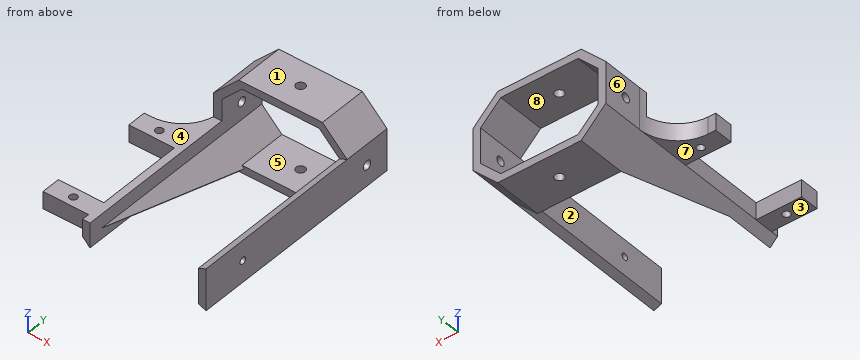
```python
from build123d import *

# Parameters (mm, degrees)
BOSS_EXTRUDE1_DEPTH = 13
BOSS_EXTRUDE2_DEPTH = 46
SKETCH8_R           = 0.9
CUT_EXTRUDE1_DEPTH  = 10
SKETCH9_R           = 1.2
CUT_EXTRUDE2_DEPTH  = 40
SKETCH10_R          = 1.2
CUT_EXTRUDE3_DEPTH  = 50
BOSS_EXTRUDE3_DEPTH = 43
SKETCH12_W          = 4.508561795
SKETCH12_H          = 5
BOSS_EXTRUDE4_DEPTH = 12
SKETCH14_R          = 1
CUT_EXTRUDE4_DEPTH  = 30
BOSS_EXTRUDE5_DEPTH = 2
FILLET3_R           = 10
BOSS_EXTRUDE6_DEPTH = 46
SKETCH8_2_R         = 0.9
CUT_EXTRUDE5_DEPTH  = 30


with BuildPart() as part:
    # Sketch1 → Boss-Extrude1 (new body)
    with BuildSketch(Plane(origin=(0, 0, 0), x_dir=(1, 0, 0), z_dir=(0, 1, 0))):
        Polygon((-7.31986533, -4.491438205), (-0.828427125, 2), (21.188696525, 2), (27.68013467, -4.491438145), (27.68013467, -15.508561795), (21.188696464, -22), (-0.828427125, -22), (-7.31986533, -15.508561795), align=None)
        Polygon((0, 0), (20.3602694, 0), (25.68013467, -5.31986527), (25.68013467, -14.68013467), (20.36026934, -20), (0, -20), (-5.31986533, -14.68013467), (-5.31986533, -5.31986533), align=None, mode=Mode.SUBTRACT)
    extrude(amount=BOSS_EXTRUDE1_DEPTH)

    # Sketch7 → Boss-Extrude2 (add)
    with BuildSketch(Plane.XZ):
        with BuildLine():
            ThreePointArc((27.68013467, 12.696190421), (26.68013467, 13.696190421), (25.68013467, 12.696190421))
            Line((25.68013467, 12.696190421), (25.68013467, 7.303809579))
            ThreePointArc((25.68013467, 7.303809579), (26.68013467, 6.303809579), (27.68013467, 7.303809579))
            Line((27.68013467, 7.303809579), (27.68013467, 12.696190421))
        make_face()
    extrude(amount=BOSS_EXTRUDE2_DEPTH)

    # Sketch8 → Cut-Extrude1 (cut)
    with BuildSketch(Plane(origin=(27.68013467, 0, 0), x_dir=(0, 0, -1), z_dir=(1, 0, 0))):
        with Locations((-10.196190421, -34)):
            Circle(SKETCH8_R)
    extrude(amount=-CUT_EXTRUDE1_DEPTH, mode=Mode.SUBTRACT)

    # Sketch9 → Cut-Extrude2 (cut)
    with BuildSketch(Plane.XY.offset(22)):
        with Locations((10.171572875, 6.5)):
            Circle(SKETCH9_R)
    extrude(amount=-CUT_EXTRUDE2_DEPTH, mode=Mode.SUBTRACT)

    # Sketch10 → Cut-Extrude3 (cut)
    with BuildSketch(Plane(origin=(27.68013467, 0, 0), x_dir=(0, 0, -1), z_dir=(1, 0, 0))):
        with Locations((-10, 6.5)):
            Circle(SKETCH10_R)
    extrude(amount=-CUT_EXTRUDE3_DEPTH, mode=Mode.SUBTRACT)

    # Sketch11 → Boss-Extrude3 (add)
    with BuildSketch(Plane.XZ):
        Polygon((-5.31986533, 9), (-7.31986533, 9), (-7.31986533, 4.491438205), (-5.31986533, 2.491438205), align=None)
    extrude(amount=BOSS_EXTRUDE3_DEPTH)

    # Sketch12 → Boss-Extrude4 (add)
    with BuildSketch(Plane.ZY.offset(7.31986533)):
        with Locations((6.745719103, -10.5)):
            Rectangle(SKETCH12_W, SKETCH12_H)
        with Locations((6.745719103, -38.5)):
            Rectangle(SKETCH12_W, SKETCH12_H)
    extrude(amount=BOSS_EXTRUDE4_DEPTH)

    # Sketch14 → Cut-Extrude4 (cut)
    with BuildSketch(Plane.XY.offset(9)):
        with Locations((-13.31986532, -10.5)):
            Circle(SKETCH14_R)
        with Locations((-13.31986532, -38.5)):
            Circle(SKETCH14_R)
    extrude(amount=-CUT_EXTRUDE4_DEPTH, mode=Mode.SUBTRACT)

    # Sketch17 → Boss-Extrude5 (add)
    with BuildSketch(Plane(origin=(-1.414213562, 0, -1.414213562), x_dir=(-0.7071067811865714, 0, 0.7071067811865236), z_dir=(-0.7071067811865236, 0, -0.7071067811865714))):
        Polygon((-0.828427125, 0), (8.351852825, -43), (8.351852825, 0), align=None)
    extrude(amount=-BOSS_EXTRUDE5_DEPTH)

    # Fillet3
    fillet3_edges = [part.edges().sort_by_distance(p)[0] for p in [
        (-7.31986533, -8, 6.745719103),
    ]]
    fillet(fillet3_edges, radius=FILLET3_R)

    # Sketch18 → Boss-Extrude6 (add)
    with BuildSketch(Plane.XZ):
        Polygon((27.68013467, 15.508561795), (25.68013467, 14.68013467), (25.68013467, 5.31986527), (27.68013467, 4.491438145), align=None)
    extrude(amount=BOSS_EXTRUDE6_DEPTH)

    # Sketch8<2> → Cut-Extrude5 (cut)
    with BuildSketch(Plane(origin=(27.68013467, 0, 0), x_dir=(0, 0, -1), z_dir=(1, 0, 0))):
        with Locations((-10.196190421, -34)):
            Circle(SKETCH8_2_R)
    extrude(amount=-CUT_EXTRUDE5_DEPTH, mode=Mode.SUBTRACT)


solid = part.part
```
Can you work these out from the model? Positions are in its coordinate system, mm. Face numbers are marked on the shaded views. A direction names the side the tool comes from. Give positions to 0.01 mm unless a question says otherwise; leave off trailing zeros. Write each loop counter-clockwise with the first axis right and the second up, starting at its lowest first coordinate (ties: lowest second). Pieces come first, ordered by that corner, then holes. Notation, with made-up numbers: (85.25, -13.5) -> (101.25, -13.5) arc R15 ccw to (101.25, -7.5) -> close; hole circle Ø10 at (-38, 18.25). An arc over 180 degrees is marked (long way). One line per item, written item: value.
Q1. We'd pull the mould along Z, two halves only. Please class the marked faces 5, 6, 7 and 8: +Z half, -Z half, draft (parallel to the pull), parting line (faces both ways), or undercut.
Results found:
face 5: undercut
face 6: draft
face 7: -Z half
face 8: undercut
Q2. Imagine slicing it at B-B on x = 4.5. Please give me the cut outline in (y, z), and give its area (3 significant figures).
Results found:
outline: (0, -2) -> (13, -2) -> (13, 0) -> (0, 0) -> close; (0, 20) -> (13, 20) -> (13, 22) -> (0, 22) -> close
area: 52.0 mm^2
Q3. Imagine slicing it at C-C on z = 17.75. Please give me the cut outline in (x, y).
Results found:
outline: (-5.08, 0) -> (-2.25, 0) -> (-2.25, 13) -> (-5.08, 13) -> close; (22.61, 0) -> (25.44, 0) -> (25.44, 13) -> (22.61, 13) -> close
Q4. Imagine slicing it at D-D on z = 10. Please give me the cut outline in (x, y).
Results found:
outline: (-7.52, 0) -> (-5.32, 0) -> (-5.32, 5.3) -> (-7.32, 5.3) -> (-7.32, 2) arc R10 cw to start; (-7.32, 7.7) -> (-5.32, 7.7) -> (-5.32, 13) -> (-7.32, 13) -> close; (25.68, -46) -> (27.68, -46) -> (27.68, -34.88) -> (25.68, -34.88) -> close; (25.68, -33.12) -> (27.68, -33.12) -> (27.68, 5.3) -> (25.68, 5.3) -> close; (25.68, 7.7) -> (27.68, 7.7) -> (27.68, 13) -> (25.68, 13) -> close
Q5. Which directions (+Z, -Z, +X, -X, +Y, -Y) give clear straight access to the entire face, cutting with the end or side of a thin tool? Please do the marked faces 1, 2, 3 and 4.
Results found:
face 1: +Z, +X, -X, +Y, -Y
face 2: +Y, -Y
face 3: -Z, -X, +Y, -Y
face 4: +Z, -X, -Y
Q6. Please list where these lines run through material, in increasing order: line 1 (X direction, y = -13.5, z = 6.5); line 2 (X direction, y = -3, z = 8.25); line 3 (Z direction, x = -5, y = 6). Write a range as [from, to].
Results found:
line 1: x = [-7.32, -5.32], [25.68, 27.68]
line 2: x = [-8.66, -5.32], [25.68, 27.68]
line 3: z = [2.17, 5], [15, 17.83]
Q7. For P1, Ø3, axis at y = 6.5, z = 10, coming from the -X side; P2, Ø3.5, axis at x = -16, z = 7, coming from the +Y side; P3, Ø1, axis at x = -18.5, z = 6.5, coming from the +Y side; P4, Ø3, axis at x = 20.5, z = 15, coming from the -Y side, each with a flat end and sliding along its axis, tell me the tip position at first contact or that it passes through.
Results found:
P1: stops at x = -7.32
P2: stops at y = -7.52
P3: stops at y = -8
P4: passes through
Q8. Imagine slicing it at A-A on y = 6.5. Give the number of separate pieces and of enclosed holes in the cut face, and give its area (3 significant figures).
Results found:
separate pieces: 4
enclosed holes: 0
area: 173 mm^2
